Here's how the part is built. I have some questions about the finished solid (model axes, mm). Face numbers are marked on the shaded views. A direction names the side the tool comes from. Round coordinates to 2 decimals unless told otherwise and drop trailing zeros. Order: outer loops, then holes, each group sorted by start corner. A loop starts at its lowest first (then second) coordinate and runs counter-clockwise, first axis right, second up. Notation, with made-up numbers: (12, 36.5) -> (45, 36.5) arc R20 ccw to (45, 41.5) -> close; hole circle Ø2 at (21.25, 83.5). An arc over 180 degrees is marked (long way). Use a Markdown table: item, result. Add a question column.
(1) I want a section at B-B, the plane z = 5. Please give me the cut outline in (x, y), then the cut area to 3 significant figures.
(2) If I drill on probe 1 along X at (y, z) = (16.5, 1); probe 2 along Y at (x, z) = (9, 4.5); probe 3 along X at (y, z) = (13, 0.75), over which ranges is the centre line in solid material (lowest first)?
(3) On a 3-axis mill with a long thin cutter (end or side, diameter ignored), from which of +Z, -Z, +X, -X, +Y, -Y can I reach the whole of each face in a straight line? I mean the marked faces 4 and 5. Say none if no direction works.
(4) I want a section at C-C, the plane x = 0. Please give me the cut outline in (y, z).
(5) I want a section at D-D, the plane y = 0. Please give me the cut outline in (x, z).
(6) I'm going to push flat-ended pins straight in: P1, Ø4, axis at y = 2, z = 1, coming from the +X side; P2, Ø8, axis at x = 16.5, y = -0.5, coming from the +Z side; P3, Ø6, axis at x = 11.5, z = 8, coming from the -Y side; P4, Ø1, axis at x = 2.5, z = 4.5, coming from the -Y side. Where does each tip first touch, or does it pass through?
(7) I want a section at A-A, the plane x = 17.5. Please give me the cut outline in (y, z) (3 decimals), then the cut area to 3 significant figures.
(8) Thinking about a two-plate mould opening in Y: for the marked faces 1, 2 and 3, which applies, pulls with the +Y half, pulls with the -Y half, needs draft (parallel to the pull), parting line crosses it, or undercut?
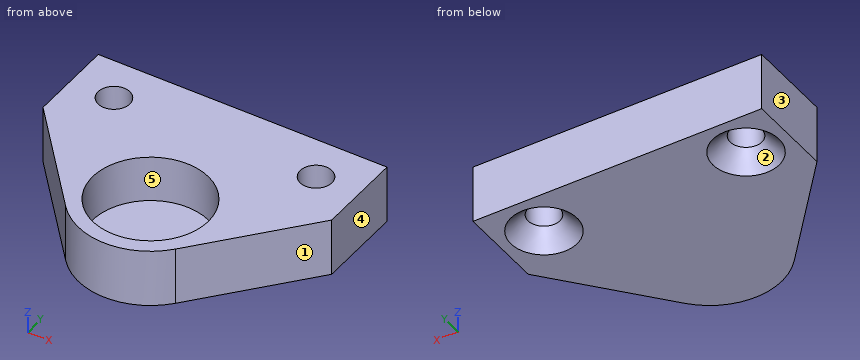
from build123d import *

# Parameters (mm, degrees)
AUFSATZ_LINEAR_AUSTRAGEN1_DEPTH                      = 10
SKIZZE2_R                                            = 10
SCHNITT_LINEAR_AUSTRAGEN1_DEPTH                      = 8
FORMSENKUNG_F_R_M5_SENKSCHRAUBE_MIT_INNE_D           = 5.5
FORMSENKUNG_F_R_M5_SENKSCHRAUBE_MIT_INNE_DEPTH       = 10
FORMSENKUNG_F_R_M5_SENKSCHRAUBE_MIT_INNE_CSINK_D     = 11.47
FORMSENKUNG_F_R_M5_SENKSCHRAUBE_MIT_INNE_CSINK_ANGLE = 90


with BuildPart() as part:
    # Skizze1 → Aufsatz-Linear austragen1 (new body)
    with BuildSketch(Plane.XY):
        with BuildLine():
            Line((-9.499737937, -8.124344843), (-25, 10))
            Line((-25, 10), (-25, 25))
            Line((-25, 25), (25, 25))
            Line((25, 25), (25, 10))
            Line((25, 10), (9.499737937, -8.124344843))
            ThreePointArc((9.499737937, -8.124344843), (0, -12.5), (-9.499737937, -8.124344843))
        make_face()
    extrude(amount=AUFSATZ_LINEAR_AUSTRAGEN1_DEPTH)

    # Skizze2 → Schnitt-Linear austragen1 (cut)
    with BuildSketch(Plane.XY.offset(10)):
        Circle(SKIZZE2_R)
    extrude(amount=-SCHNITT_LINEAR_AUSTRAGEN1_DEPTH, mode=Mode.SUBTRACT)

    # Formsenkung für M5 Senkschraube mit Innensechskant1
    with Locations(Plane(origin=(0, 0, 0), x_dir=(-1, 0, 0), z_dir=(0, 0, -1))):
        with Locations((-17.5, 17.499100788), (17.5, 17.499100788)):
            CounterSinkHole(FORMSENKUNG_F_R_M5_SENKSCHRAUBE_MIT_INNE_D / 2, FORMSENKUNG_F_R_M5_SENKSCHRAUBE_MIT_INNE_CSINK_D / 2, depth=FORMSENKUNG_F_R_M5_SENKSCHRAUBE_MIT_INNE_DEPTH, counter_sink_angle=FORMSENKUNG_F_R_M5_SENKSCHRAUBE_MIT_INNE_CSINK_ANGLE)


solid = part.part
Taken from the geometry:
| question | item | result |
|---|---|---|
| 1 | outline | (-25, 10) -> (-9.5, -8.12) arc R12.5 ccw to (9.5, -8.12) -> (25, 10) -> (25, 25) -> (-25, 25) -> close; hole circle Ø5.5 at (-17.5, 17.5); hole circle Ø20 at (0, 0); hole circle Ø5.5 at (17.5, 17.5) |
| 1 | area | 1,070 mm2 |
| 2 | probe 1 | x = -25 to -22.13, -12.87 to 12.87, 22.13 to 25 |
| 2 | probe 2 | y = -8.67 to -4.36, 4.36 to 25 |
| 2 | probe 3 | x = -25 to -19.65, -15.35 to 15.35, 19.65 to 25 |
| 3 | face 4 | +Z, -Z, +X, +Y, -Y |
| 3 | face 5 | +Z |
| 4 | outline | (-12.5, 0) -> (25, 0) -> (25, 10) -> (10, 10) -> (10, 2) -> (-10, 2) -> (-10, 10) -> (-12.5, 10) -> close |
| 5 | outline | (-16.45, 0) -> (16.45, 0) -> (16.45, 10) -> (10, 10) -> (10, 2) -> (-10, 2) -> (-10, 10) -> (-16.45, 10) -> close |
| 6 | P1 | stops at x = 19.87 |
| 6 | P2 | stops at z = 10 |
| 6 | P3 | stops at y = -9.17 |
| 6 | P4 | stops at y = -12.34 |
| 7 | outline | (1.23, 0) -> (11.764, 0) -> (14.749, 2.985) -> (14.749, 10) -> (1.23, 10) -> close; (20.249, 2.985) -> (23.234, 0) -> (25, 0) -> (25, 10) -> (20.249, 10) -> close |
| 7 | area | 174 mm2 |
| 8 | face 1 | pulls with the -Y half |
| 8 | face 2 | undercut |
| 8 | face 3 | needs draft |
